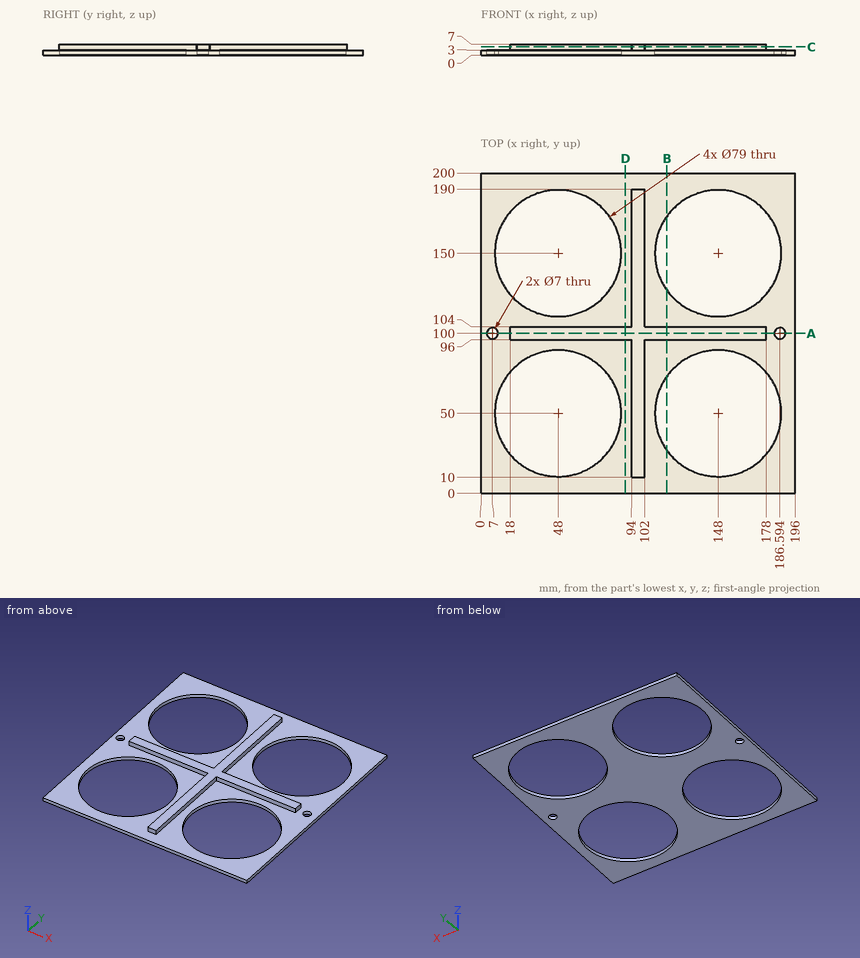
Print and shaded views of the part. All mm, measured from the part's lowest x, y and z. Give positions to 0.01 mm unless a question says otherwise; leave off trailing zeros. Loops run counter-clockwise (first coordinate to the right, second up) from the corner with the lowest first, then second, coordinate; pieces in that order, holes last. Notation, with made-up numbers: (0, 69.25) -> (13, 69.25) arc R31 cw to (13, 101.25) -> close; hole circle Ø6 at (0.5, 34.25). An arc over 180 degrees is marked (long way). Answer in a Markdown table with one row per item.
Item 1: Slice it at A-A on y = 100. Write the cut outline in (x, z).
Findings below:
| item | result |
|---|---|
| outline | (0, 0) -> (3.5, 0) -> (3.5, 3) -> (0, 3) -> close; (10.5, 0) -> (183.09, 0) -> (183.09, 3) -> (178, 3) -> (178, 7) -> (18, 7) -> (18, 3) -> (10.5, 3) -> close; (190.09, 0) -> (196, 0) -> (196, 3) -> (190.09, 3) -> close |
Item 2: Slice it at C-C on z = 5.25. Write the cut outline in (x, y).
Findings below:
| item | result |
|---|---|
| outline | (18, 96) -> (94, 96) -> (94, 10) -> (102, 10) -> (102, 96) -> (178, 96) -> (178, 104) -> (102, 104) -> (102, 190) -> (94, 190) -> (94, 104) -> (18, 104) -> close |
Item 3: Slice it at D-D on x = 90. Write the cut outline in (y, z), plus the area to 3 significant figures.
Findings below:
| item | result |
|---|---|
| outline | (0, 0) -> (200, 0) -> (200, 3) -> (104, 3) -> (104, 7) -> (96, 7) -> (96, 3) -> (0, 3) -> close |
| area | 632 mm² |
Item 4: Probe line 1 along Y through (x, z) = (48, 1.7); line 2 along X through (y, z) = (152, 2.25); line 3 along X through (y, z) = (49, 2.25). List the from-to ranges inside material, lowest first. Write a range as [from, to].
Findings below:
| item | result |
|---|---|
| line 1 | y = [0, 10.5], [89.5, 110.5], [189.5, 200] |
| line 2 | x = [0, 8.55], [87.45, 108.55], [187.45, 196] |
| line 3 | x = [0, 8.51], [87.49, 108.51], [187.49, 196] |
Item 5: Flat gauge pins, fed straight in: P1, Ø3, axis at x = 113.5, z = 6, coming from the -Y side; P2, Ø1, axis at x = 115, y = 122.5, coming from the +Z side; P3, Ø3, axis at y = 100.5, z = 5, coming from the +X side. Where does each tip first touch, or does it go through?
Findings below:
| item | result |
|---|---|
| P1 | stops at y = 96 |
| P2 | stops at z = 3 |
| P3 | stops at x = 178 |
Item 6: Slice it at B-B on x = 116. Write the cut outline in (y, z), plus the area to 3 significant figures.
Findings below:
| item | result |
|---|---|
| outline | (0, 0) -> (26.84, 0) -> (26.84, 3) -> (0, 3) -> close; (73.16, 0) -> (126.84, 0) -> (126.84, 3) -> (104, 3) -> (104, 7) -> (96, 7) -> (96, 3) -> (73.16, 3) -> close; (173.16, 0) -> (200, 0) -> (200, 3) -> (173.16, 3) -> close |
| area | 354 mm² |
